Geometry check sheet. Reference: the model listing, model coordinates, mm. A direction names the side the tool comes from. Give positions to 0.01 mm unless a question says otherwise; leave off trailing zeros. Loops run counter-clockwise (first coordinate to the right, second up) from the corner with the lowest first, then second, coordinate; pieces in that order, holes last. Notation, with made-up numbers: (85.25, 26) -> (112.25, 26) arc R13 ccw to (112.25, 41) -> close; hole circle Ø10 at (-29, 27). An arc over 180 degrees is marked (long way). Write each question's results on one line, items separated by ' | '. Start each with the question number.
1) Set-up check for faces 1 (the face through (0, 13, 0)), 2 (the face through (12.832, 11.661, 16.015)): record each of +Z, -Z, +X, -X, +Y, -Y from which the full face is reachable in a straight line by a thin tool's end or side.
2) Depth check by flat-ended pin: pin 1 (4 mm diameter, centred on x = 7, y = 9, fed in from -Z); pin 2 (6 mm diameter, centred on y = 14.5, z = -3.5, fed in from +X); pin 3 (17 mm diameter, centred on x = -5.5, z = 10.5, fed in from +Y). Enter the tip coordinate at first touch or a pass-through.
3) Sectioned sample at D-D on x = 0. Record the cut outline in (y, z) (3 decimals), then the cut area to 3 significant figures.
4) Scan lines: line 1 (Z direction, x = 10.95, y = 10.75); line 2 (Z direction, x = -21.9, y = 14.75) (3 decimals); line 3 (Y direction, x = 1.5, z = 14.5). Record each from-to range of solid material in increasing order. Write a range as from..to.
5) Sectioned sample at A-A on y = 19.5. Record the cut outline in (x, z) (3 decimals).
6) Draft check along Z on faces 3 (the face through (-16.84, 17.93, -3.88)), 4 (the face through (10, 23, 23)), 5 (the face through (16.009, 17.93, -22.845)). Enter one of: pulls with the +Z half, pulls with the -Z half, needs draft (parallel to the pull), parting line crosses it, or undercut.
7) Sectioned sample at C-C on x = -21.9. Record the cut outline in (y, z) (3 decimals).
8) Sectioned sample at B-B on x = 10.95. Record the cut outline in (y, z).
```python
from build123d import *

# Parameters (mm, degrees)
SKETCH3_R           = 28.275
BOSS_EXTRUDE1_DEPTH = 13
SKETCH4_R           = 6.375
BOSS_EXTRUDE2_DEPTH = 10
D_GAGEMENT_M1_61_D  = 7


with BuildPart() as part:
    # Sketch3 → Boss-Extrude1 (new body)
    with BuildSketch(Plane(origin=(0, 0, 0), x_dir=(1, 0, 0), z_dir=(0, 1, 0))):
        with Locations(Location((0, 0, 0), (0, 0, 90))):
            Circle(SKETCH3_R)
    extrude(amount=BOSS_EXTRUDE1_DEPTH)

    # Sketch4 → Boss-Extrude2 (add)
    with BuildSketch(Plane(origin=(0, 13, 0), x_dir=(1, 0, 0), z_dir=(0, 1, 0))):
        with Locations(Location((-21.9, 0, 0), (0, 0, 179.999635348))):
            Circle(SKETCH4_R)
        with Locations(Location((10.95, 18.965956343, 0), (0, 0, 59.999635366))):
            Circle(SKETCH4_R)
        with Locations(Location((10.95, -18.965956343, 0), (0, 0, 299.999635366))):
            Circle(SKETCH4_R)
    extrude(amount=BOSS_EXTRUDE2_DEPTH)

    # Dégagement M1.61 (through all)
    with Locations(Plane(origin=(0, 0, 0), x_dir=(-1, 0, 0), z_dir=(0, -1, 0))):
        with Locations((21.9, 0), (-10.95, 18.965956343), (-10.95, -18.965956343)):
            Hole(D_GAGEMENT_M1_61_D / 2)


solid = part.part
```
Result:
1) face 1: +Y | face 2: +Y, -Y
2) pin 1: z = -27.83 | pin 2: x = 28.26 | pin 3: y = 13
3) outline: (0, -28.275) -> (13, -28.275) -> (13, 28.275) -> (0, 28.275) -> close | area: 735 mm^2
4) line 1: -26.07..-22.47, -15.47..15.47, 22.47..26.07 | line 2: -6.375..-3.5, 3.5..6.375 | line 3: 0..13
5) outline: circle Ø12.75 at (-21.9, 0); circle Ø12.75 at (10.95, -18.966); circle Ø12.75 at (10.95, 18.966); hole circle Ø7 at (-21.9, 0); hole circle Ø7 at (10.95, -18.966); hole circle Ø7 at (10.95, 18.966)
6) face 3: parting line crosses it | face 4: needs draft | face 5: undercut
7) outline: (0, -17.885) -> (13, -17.885) -> (13, -6.375) -> (23, -6.375) -> (23, -3.5) -> (0, -3.5) -> close; (0, 3.5) -> (23, 3.5) -> (23, 6.375) -> (13, 6.375) -> (13, 17.885) -> (0, 17.885) -> close
8) outline: (0, -26.07) -> (13, -26.07) -> (13, -25.34) -> (23, -25.34) -> (23, -22.47) -> (0, -22.47) -> close; (0, -15.47) -> (23, -15.47) -> (23, -12.59) -> (13, -12.59) -> (13, 12.59) -> (23, 12.59) -> (23, 15.47) -> (0, 15.47) -> close; (0, 22.47) -> (23, 22.47) -> (23, 25.34) -> (13, 25.34) -> (13, 26.07) -> (0, 26.07) -> close
